Print and shaded views of the part. All mm, measured from the part's lowest x, y and z. Coordinates: 2 decimals unless noted, no trailing zeros. Order: outer loops, then holes, each group sorted by start corner. A loop starts at its lowest first (then second) coordinate and runs counter-clockwise, first axis right, second up. Notation, with made-up numbers: (5.5, -30) -> (32.5, -30) arc R22 cw to (32.5, -2) -> close; hole circle Ø10 at (5, 46.25). An arc over 180 degrees is marked (long way). Write item = value, one per line. Start each with the question number.
Q1. Cut at C-C, the plane x = 56.5. List the corners of the cut face in (y, z), plus the area to 3 significant figures.
Q2. Cut at B-B, the plane z = 3. List the corners of the cut face in (x, y).
Q3. Flat gauge pins, fed straight in: pin 1 (4.5 mm diameter, centred on y = 31.5, z = 13.5, fed in from -X); pin 2 (4 mm diameter, centred on y = 20.5, z = 1.5, fed in from +X); pin 3 (0.8 mm diameter, centred on x = 32.5, z = 15.5, fed in from +Y). Where does each tip first touch, or does it go through?
Q4. Cut at A-A, the plane z = 13.5. List the corners of the cut face in (x, y), plus the area to 3 significant figures.
Q5. Wall check: line 1 (Y direction, x = 33, z = 11.5); line 2 (X direction, y = 57.5, z = 2.5); line 3 (Z direction, x = 11, y = 27.5). Give the ranges that are in metal, low to high. Write a range as from..to.
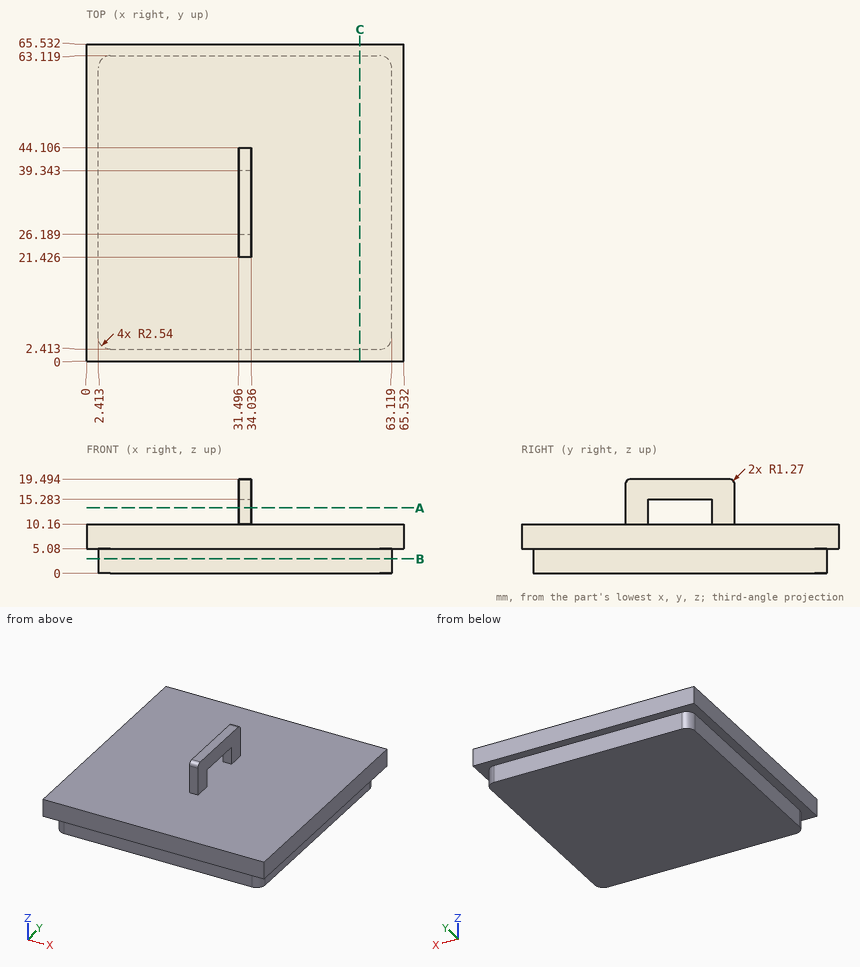
Here are the results:
q1.outline = (0, 5.08) -> (2.41, 5.08) -> (2.41, 0) -> (63.12, 0) -> (63.12, 5.08) -> (65.53, 5.08) -> (65.53, 10.16) -> (0, 10.16) -> close
q1.area = 641 mm²
q2.outline = (2.41, 4.95) arc R2.54 ccw to (4.95, 2.41) -> (60.58, 2.41) arc R2.54 ccw to (63.12, 4.95) -> (63.12, 60.58) arc R2.54 ccw to (60.58, 63.12) -> (4.95, 63.12) arc R2.54 ccw to (2.41, 60.58) -> close
q3.pin_1 = 31.5
q3.pin_2 = 63.12
q3.pin_3 = 44.11
q4.outline = (31.5, 21.43) -> (34.04, 21.43) -> (34.04, 26.19) -> (31.5, 26.19) -> close; (31.5, 39.34) -> (34.04, 39.34) -> (34.04, 44.11) -> (31.5, 44.11) -> close
q4.area = 24.2 mm²
q5.line_1 = 21.43..26.19, 39.34..44.11
q5.line_2 = 2.41..63.12
q5.line_3 = 0..10.16
